For this review, take the finished solid that the model builds, in its own axes (mm). Face numbers are marked on the shaded views. Round coordinates to 2 decimals unless told otherwise and drop trailing zeros. Write each loop counter-clockwise with the first axis right and the second up, starting at its lowest first coordinate (ties: lowest second). Pieces come first, ordered by that corner, then holes. Notation, with made-up numbers: (35, 87) - (55, 87) arc R21 ccw to (55, 98) - close; hole circle Ø9 at (76, 50). An arc over 180 degrees is marked (long way). Answer in a Markdown table with one row per item. Add a question column.
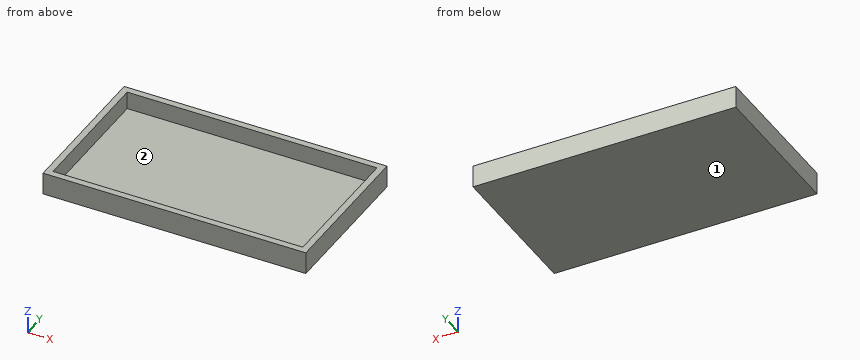
from build123d import *

# Parameters (mm, degrees)
F0_W          = 201.395
F0_H          = 116.729
F1_DEPTH      = 8.515
F2_W          = 191.395
F2_H          = 106.729
F3_DEPTH      = 8.515
F3_DEPTH_BACK = 5


with BuildPart() as f1:
    # F0 (on Top) → F1 (new body, symmetric)
    with BuildSketch(Plane.XY):
        with Locations((95.6975, -53.3645)):
            Rectangle(F0_W, F0_H)
    extrude(amount=F1_DEPTH, both=True)

    # F2 (on Top) → F3 (cut, two sides)
    with BuildSketch(Plane.XY) as f3_sk:
        with Locations((95.6975, -53.3645)):
            Rectangle(F2_W, F2_H)
    extrude(amount=F3_DEPTH, mode=Mode.SUBTRACT)
    extrude(f3_sk.sketch, amount=-F3_DEPTH_BACK, mode=Mode.SUBTRACT)


solid = f1.part
Q1. Add section B-B on y = -52. State the section outline as (x, z) points (3 decimals).
Q2. Draft analysis for pull direction X (two halves, no side actions). For the marked faces 1 and 2, state which applies: released by +X, released by -X, zero draft, split by the parting line, or undercut.
Q3. To check wall thickness, follow probe 1 along X at (y, z) = (-96, 7) (3 decimals); probe 2 along Y at (x, z) = (32, -4.75); probe 3 along Z at (x, y) = (33, -81) (3 decimals). State the ranges of each line that lie inside material, in increasing order.
Q4. Add section C-C on x = 173. State the section outline as (y, z) points (3 decimals).
Q5. Add section A-A on z = 1.5. State the section outline as (x, y) points (3 decimals).
Answer sheet:
| question | item | result |
|---|---|---|
| 1 | outline | (-5, -8.515) - (196.395, -8.515) - (196.395, 8.515) - (191.395, 8.515) - (191.395, -5) - (0, -5) - (0, 8.515) - (-5, 8.515) - close |
| 2 | face 1 | zero draft |
| 2 | face 2 | undercut |
| 3 | probe 1 | x = -5 to 0, 191.395 to 196.395 |
| 3 | probe 2 | y = -111.73 to -106.73, 0 to 5 |
| 3 | probe 3 | z = -8.515 to -5 |
| 4 | outline | (-111.729, -8.515) - (5, -8.515) - (5, 8.515) - (0, 8.515) - (0, -5) - (-106.729, -5) - (-106.729, 8.515) - (-111.729, 8.515) - close |
| 5 | outline | (-5, -111.729) - (196.395, -111.729) - (196.395, 5) - (-5, 5) - close; hole (0, -106.729) - (191.395, -106.729) - (191.395, 0) - (0, 0) - close |
